For this review, take the finished solid that the model builds, in its own axes (mm). A direction names the side the tool comes from. Coordinates: 2 decimals unless noted, no trailing zeros.
```python
from build123d import *

# Parameters (mm, degrees)
F0_R      = 1.5
F1_DEPTH  = 1.5
F2_W      = 80
F2_H      = 87
F2_W_2    = 1.5
F2_H_2    = 80
F2_H_3    = 2
F3_DEPTH  = 22.5
F4_START  = 24
F4_DEPTH  = 1.5
F6_START  = -87
F5_W      = 68
F5_H      = 18
F6_DEPTH  = 5
F7_DEPTH  = 16
F8_R      = 10
F9_R      = 2
F10_R     = 4.75
F10_R_2   = 4
F11_DEPTH = 2
F10_R_3   = 1.75
F12_DEPTH = 10
F13_START = 10
F13_DEPTH = 5.5


# Not quite as in the source:
# - a fillet or chamfer that OpenCascade refuses, or shapes differently, is made with other operations: its cross-section is extruded or revolved along the edge and cut away or added


with BuildPart() as f1:
    # F0 (on Top) → F1 (new body)
    with BuildSketch(Plane.XY):
        Polygon((30, 43.5), (-40, 43.5), (-40, -43.5), (40, -43.5), (40, 27.5), (40, 43.5), align=None)
        with Locations((-36.5, -36.5)):
            Circle(F0_R, mode=Mode.SUBTRACT)
        with Locations((36.5, -36.5)):
            Circle(F0_R, mode=Mode.SUBTRACT)
        with Locations((-36.5, 36.5)):
            Circle(F0_R, mode=Mode.SUBTRACT)
        Polygon((30, 27.5), (35.5, 27.5), (35.5, -27.5), (30, -27.5), (30, -40), (-30, -40), (-30, -27.5), (-35.5, -27.5), (-35.5, 27.5), (-30, 27.5), (-30, 40), (30, 40), align=None, mode=Mode.SUBTRACT)
        with Locations((36.5, 36.5)):
            Circle(F0_R, mode=Mode.SUBTRACT)
    extrude(amount=F1_DEPTH)

    # F2 (on face) → F3 (join)
    with BuildSketch(Plane.XY.offset(1.5)):
        Rectangle(F2_W, F2_H)
        Polygon((-38.5, -42), (-38.5, 42), (-30.5, 42), (-29, 42), (-22, 42), (-20.5, 42), (-13.5, 42), (-12, 42), (-5, 42), (-3.5, 42), (3.5, 42), (5, 42), (12, 42), (13.5, 42), (20.5, 42), (22, 42), (29, 42), (30.5, 42), (38.5, 42), (38.5, -42), (30.5, -42), (29, -42), (22, -42), (20.5, -42), (13.5, -42), (12, -42), (5, -42), (3.5, -42), (-3.5, -42), (-5, -42), (-12, -42), (-13.5, -42), (-20.5, -42), (-22, -42), (-29, -42), (-30.5, -42), align=None, mode=Mode.SUBTRACT)
        Polygon((-30, 27.5), (-30.5, 27.5), (-30.5, -27.5), (-30, -27.5), (-30, -40), (-29, -40), (-29, 40), (-30, 40), align=None)
        Polygon((-29, 42), (-30.5, 42), (-30.5, 27.5), (-30, 27.5), (-30, 40), (-29, 40), align=None)
        with Locations((-21.25, 0)):
            Rectangle(F2_W_2, F2_H_2)
        with Locations((-12.75, 0)):
            Rectangle(F2_W_2, F2_H_2)
        with Locations((-4.25, 0)):
            Rectangle(F2_W_2, F2_H_2)
        with Locations((4.25, 0)):
            Rectangle(F2_W_2, F2_H_2)
        with Locations((12.75, 0)):
            Rectangle(F2_W_2, F2_H_2)
        with Locations((21.25, 0)):
            Rectangle(F2_W_2, F2_H_2)
        Polygon((30, 40), (29, 40), (29, -40), (30, -40), (30, -27.5), (30.5, -27.5), (30.5, 27.5), (30, 27.5), align=None)
        Polygon((29, -40), (29, -42), (30.5, -42), (30.5, -27.5), (30, -27.5), (30, -40), align=None)
        Polygon((30.5, 42), (29, 42), (29, 40), (30, 40), (30, 27.5), (30.5, 27.5), align=None)
        Polygon((-30.5, -27.5), (-30.5, -42), (-29, -42), (-29, -40), (-30, -40), (-30, -27.5), align=None)
        with Locations((21.25, -41)):
            Rectangle(F2_W_2, F2_H_3)
        with Locations((12.75, -41)):
            Rectangle(F2_W_2, F2_H_3)
        with Locations((-4.25, -41)):
            Rectangle(F2_W_2, F2_H_3)
        with Locations((4.25, -41)):
            Rectangle(F2_W_2, F2_H_3)
        with Locations((-12.75, -41)):
            Rectangle(F2_W_2, F2_H_3)
        with Locations((-21.25, -41)):
            Rectangle(F2_W_2, F2_H_3)
        with Locations((21.25, 41)):
            Rectangle(F2_W_2, F2_H_3)
        with Locations((12.75, 41)):
            Rectangle(F2_W_2, F2_H_3)
        with Locations((4.25, 41)):
            Rectangle(F2_W_2, F2_H_3)
        with Locations((-4.25, 41)):
            Rectangle(F2_W_2, F2_H_3)
        with Locations((-12.75, 41)):
            Rectangle(F2_W_2, F2_H_3)
        with Locations((-21.25, 41)):
            Rectangle(F2_W_2, F2_H_3)
    extrude(amount=F3_DEPTH)

    # F0 (on Top) → F4 (join)
    with BuildSketch(Plane.XY.offset(F4_START)):
        Polygon((30, 43.5), (-40, 43.5), (-40, -43.5), (40, -43.5), (40, 27.5), (40, 43.5), align=None)
        with Locations((-36.5, -36.5)):
            Circle(F0_R, mode=Mode.SUBTRACT)
        with Locations((36.5, -36.5)):
            Circle(F0_R, mode=Mode.SUBTRACT)
        with Locations((-36.5, 36.5)):
            Circle(F0_R, mode=Mode.SUBTRACT)
        Polygon((30, 27.5), (35.5, 27.5), (35.5, -27.5), (30, -27.5), (30, -40), (-30, -40), (-30, -27.5), (-35.5, -27.5), (-35.5, 27.5), (-30, 27.5), (-30, 40), (30, 40), align=None, mode=Mode.SUBTRACT)
        with Locations((36.5, 36.5)):
            Circle(F0_R, mode=Mode.SUBTRACT)
    extrude(amount=F4_DEPTH)

    # F5 (on face) → F6 (join)
    with BuildSketch(Plane(origin=(0, 43.5, 0), x_dir=(-1, 0, 0), z_dir=(0, 1, 0)).offset(F6_START)):
        with Locations((0, 12.75)):
            Rectangle(F5_W, F5_H)
    extrude(amount=-F6_DEPTH)

    # F5 (on face) → F7 (join)
    with BuildSketch(Plane(origin=(0, 43.5, 0), x_dir=(-1, 0, 0), z_dir=(0, 1, 0))):
        with Locations((0, 12.75)):
            Rectangle(F5_W, F5_H)
    extrude(amount=F7_DEPTH)

    # F8
    f8_edges = [f1.edges().sort_by_distance(p)[0] for p in [
        (34, 59.5, 12.75),
        (-34, 59.5, 12.75),
    ]]
    fillet(f8_edges, radius=F8_R)

    # F9
    f9_edges = [f1.edges().sort_by_distance(p)[0] for p in [
        (34, 46.5, 3.75),
        (31.071068, 56.571068, 3.75),
        (0, 43.5, 3.75),
        (0, 59.5, 3.75),
        (-34, 46.5, 3.75),
        (-31.071068, 56.571068, 3.75),
        (-34, 46.5, 21.75),
        (-31.071068, 56.571068, 21.75),
        (0, 43.5, 21.75),
        (0, 59.5, 21.75),
        (34, 46.5, 21.75),
        (31.071068, 56.571068, 21.75),
        (0, -48.5, 21.75),
        (34, -48.5, 12.75),
        (0, -48.5, 3.75),
        (-34, -48.5, 12.75),
        (0, -43.5, 21.75),
        (34, -43.5, 12.75),
        (0, -43.5, 3.75),
        (-34, -43.5, 12.75),
        (-34, -46, 21.75),
        (-34, -46, 3.75),
        (34, -46, 3.75),
        (34, -46, 21.75),
        (-34, 43.5, 12.75),
        (34, 43.5, 12.75),
    ]]
    fillet(f9_edges, radius=F9_R)

    # F10 (on face) → F11 (join)
    with BuildSketch(Plane.XY.offset(21.75)):
        with BuildLine():
            ThreePointArc((-30.6249429729, 53.9844320271), (-27.2809272798, 46.4086617374), (-20.75, 51.5))
            ThreePointArc((-20.75, 51.5), (-23.3056325549, 56.0058721765), (-28.4844320271, 56.1249429729))
            ThreePointArc((-28.4844320271, 56.1249429729), (-29.6568542495, 55.1568542495), (-30.6249429729, 53.9844320271))
        make_face()
        with Locations((-26, 51.5)):
            Circle(F10_R, mode=Mode.SUBTRACT)
        with Locations((-26, 51.5)):
            Circle(F10_R)
        with Locations((-26, 51.5)):
            Circle(F10_R_2, mode=Mode.SUBTRACT)
        with BuildLine():
            ThreePointArc((30.6249429729, 53.9844320271), (29.6568542495, 55.1568542495), (28.4844320271, 56.1249429729))
            ThreePointArc((28.4844320271, 56.1249429729), (21.4941278235, 48.8056325549), (31.25, 51.5))
            ThreePointArc((31.25, 51.5), (31.0913382626, 52.7809272798), (30.6249429729, 53.9844320271))
        make_face()
        with Locations((26, 51.5)):
            Circle(F10_R, mode=Mode.SUBTRACT)
        with Locations((26, 51.5)):
            Circle(F10_R)
        with Locations((26, 51.5)):
            Circle(F10_R_2, mode=Mode.SUBTRACT)
    extrude(amount=F11_DEPTH)

    # F10 (on face) → F12 (join)
    with BuildSketch(Plane.XY.offset(21.75)):
        with Locations((-26, 51.5)):
            Circle(F10_R_2)
        with Locations((-26, 51.5)):
            Circle(F10_R_3, mode=Mode.SUBTRACT)
        with Locations((26, 51.5)):
            Circle(F10_R_2)
        with Locations((26, 51.5)):
            Circle(F10_R_3, mode=Mode.SUBTRACT)
    extrude(amount=F12_DEPTH)

    # F10 (on face) → F13 (join)
    with BuildSketch(Plane.XY.offset(21.75).offset(F13_START)):
        with Locations((-26, 51.5)):
            Circle(F10_R)
        with Locations((-26, 51.5)):
            Circle(F10_R_2, mode=Mode.SUBTRACT)
        with Locations((26, 51.5)):
            Circle(F10_R)
        with Locations((26, 51.5)):
            Circle(F10_R_2, mode=Mode.SUBTRACT)
        with Locations((-26, 51.5)):
            Circle(F10_R_2)
        with Locations((-26, 51.5)):
            Circle(F10_R_3, mode=Mode.SUBTRACT)
        with Locations((26, 51.5)):
            Circle(F10_R_2)
        with Locations((26, 51.5)):
            Circle(F10_R_3, mode=Mode.SUBTRACT)
    extrude(amount=F13_DEPTH)

    # F14: fillet of radius 4 on 2 edges, made by hand

    # F14_s1 → F14_t2 (revolve, cut)
    with BuildSketch(Plane.XZ.offset(-51.5)):
        with BuildLine():
            ThreePointArc((-21.25, 33.3770166538), (-22.0877223398, 35.8265063966), (-24.25, 37.25))
            Line((-24.25, 37.25), (-21.25, 37.25))
            Line((-21.25, 37.25), (-21.25, 33.3770166538))
        make_face()
    revolve(axis=Axis((-26, 51.5, 37.25), (0, 0, 1)), mode=Mode.SUBTRACT)

    # F14_s3 → F14_t4 (revolve, cut)
    with BuildSketch(Plane.XZ.offset(-51.5)):
        with BuildLine():
            ThreePointArc((30.75, 33.3770166538), (29.9122776602, 35.8265063966), (27.75, 37.25))
            Line((27.75, 37.25), (30.75, 37.25))
            Line((30.75, 37.25), (30.75, 33.3770166538))
        make_face()
    revolve(axis=Axis((26, 51.5, 37.25), (0, 0, 1)), mode=Mode.SUBTRACT)


solid = f1.part
```
Q1. Clearance check with flat-ended pins moving along their axes: pin 1 Ø1.5 at (x, z) = (-10, 23) entering from -Y; pin 2 Ø0.8 at (x, z) = (33.5, 1) entering from +Y; pin 3 Ø3 at (x, y) = (-9, 8.5) entering from -Z; pin 4 Ø1.6 at (x, y) = (-4.5, 14) entering from -Z. State where each tip first meets the part, or that it passes through.
Ans:
pin 1: stops at y = -44.18
pin 2: stops at y = 43.5
pin 3: passes through
pin 4: stops at z = 1.5
Q2. Add section B-B (y = 30.5). Give the number of separate pieces and of enclosed holes in the cut face, then the cut area to 4 significant figures.
Ans:
separate pieces: 8
enclosed holes: 2
area: 397.5 mm2
Q3. For probe 1 along Y at (x, z) = (36.5, 24.6); probe 2 along Y at (x, z) = (26, 27.5); probe 3 along Y at (x, z) = (-33.5, 2), list the stretches that pass through material, from the lowest coordinate up.
Ans:
probe 1: y = -43.5 to -38, -35 to 35, 38 to 43.5
probe 2: y = 47.5 to 49.75, 53.25 to 55.5
probe 3: y = -43.5 to -42, 42 to 43.5
Q4. Draft analysis for pull direction Y (two halves, no side actions). For faces 4 (the flat face through (0, -48.5, 13)), 5 (the flat face through (-26, 42, 13)), 6 (the flat face through (-36, 3, 25.5)), 7 (the cylindrical face through (30.53, 52.93, 32.55)), state which applies: +Y half, -Y half, draft (parallel to the pull), parting line (faces both ways), or undercut.
Ans:
face 4: -Y half
face 5: undercut
face 6: draft
face 7: parting line
Q5. Tool access review of faces 1 (the cylindrical face through (-27.39, 50.44, 29.39)), 2 (the cylindrical face through (29.672, 55.142, 22.736)), 3 (the flat face through (17, 42, 13)): name each direction out of +Z, -Z, +X, -X, +Y, -Y from which nothing blocks a thin tool from reaching the whole face with its end or side.
Ans:
face 1: +Z
face 2: +Z, +X, +Y
face 3: none
